from build123d import *

# Parameters (mm, degrees)
F0_W     = 14
F0_H     = 2
F3_SIZE  = 0.2
F4_W     = 1.125
F4_H     = 1.5
F5_DEPTH = 15


# Not quite as in the source:
# - a fillet or chamfer that OpenCascade refuses, or shapes differently, is made with other operations: its cross-section is extruded or revolved along the edge and cut away or added


with BuildPart() as f1:
    # F0 (on Front) → F1 (revolve)
    with BuildSketch(Plane.XZ):
        with Locations((0.5, 1)):
            Rectangle(F0_W, F0_H)
        Polygon((-8.5, 0), (-6.5, 0), (-6.5, 2), (-6.5, 3.5), (-8.5, 3.5), align=None)
    revolve(axis=Axis((-0.5, 0, 0), (-1, 0, 0)))

    # F2: fillet of radius 3.5 on 1 edges, made by hand

    # F2_s1 → F2_t2 (revolve, cut)
    with BuildSketch(Plane.XZ):
        with BuildLine():
            ThreePointArc((-6.5, 3.5), (-7.9580398915, 2.2085510332), (-8.5, 0.3377223398))
            Line((-8.5, 0.3377223398), (-8.5, 3.5))
            Line((-8.5, 3.5), (-6.5, 3.5))
        make_face()
    revolve(axis=Axis((-8.5, 0, 0), (-1, 0, 0)), mode=Mode.SUBTRACT)

    # F3
    f3_edges = [f1.edges().sort_by_distance(p)[0] for p in [
        (7.5, 0, -2),
    ]]
    chamfer(f3_edges, length=F3_SIZE)

    # F4 (on face) → F5 (cut, symmetric)
    with BuildSketch(Plane.XZ):
        with Locations((-8.5627762601, 0)):
            Rectangle(F4_W, F4_H)
    extrude(amount=F5_DEPTH, both=True, mode=Mode.SUBTRACT)


solid = f1.part
Read the model definition and answer for the solid it produces. Units are mm, in the model's axes. A direction names the side the tool comes from. Give positions to 0.01 mm unless a question says otherwise; leave off trailing zeros. Write each loop counter-clockwise with the first axis right and the second up, starting at its lowest first coordinate (ties: lowest second). Pieces come first, ordered by that corner, then holes. Notation, with made-up numbers: (9, 69) - (52, 69) arc R21 cw to (52, 97) - close; hole circle Ø10 at (-1.75, 34). An arc over 180 degrees is marked (long way). Answer in a Markdown table with one row per item. Add a question column.
Item 1: Flat-ended cylindrical pins translate along their axes: P1, Ø2, axis at y = -1.5, z = -1, coming from the -X side; P2, Ø4, axis at y = -2, z = -1, coming from the +X side; P3, Ø2, axis at x = 1, y = -1.5, coming from the +Z side; P4, Ø1.2, axis at y = -1, z = 0, coming from the -X side. Find the tip coordinate at first contact, or state that the pin passes through.
Item 2: A tool of negligible diameter and unlimited length cuts with its end or side. For faces 1 (the face through (-8, 0, 0)), 2 (the face through (7.5, 0, 0)), 3 (the face through (-6.5, -2, -2)), from which of +Z, -Z, +X, -X, +Y, -Y can it reach the whole face along a straight path? Write none if from no direction.
Item 3: Find the intervals of material crossed by L1, parallel to X at y = 0.75, z = 2; L2, parallel to X at y = 0.25, z = -3; L3, parallel to Y at x = -2.5, z = 0.25, in increasing order.
Item 4: Section A-A, the plane x = 1 is taken. Write down the section's boundary in (y, z).
Recorded:
| question | item | result |
|---|---|---|
| 1 | P1 | stops at x = -8.45 |
| 1 | P2 | stops at x = 7.5 |
| 1 | P3 | stops at z = 1.94 |
| 1 | P4 | stops at x = -8 |
| 2 | face 1 | -X, +Y, -Y |
| 2 | face 2 | +Z, -Z, +X, +Y, -Y |
| 2 | face 3 | +X |
| 3 | L1 | x = -8 to -6.5 |
| 3 | L2 | x = -7.26 to -6.5 |
| 3 | L3 | y = -1.98 to 1.98 |
| 4 | outline | circle Ø4 at (0, 0) |
